from build123d import *

# Parameters (mm, degrees)
SKETCH1_W           = 27
SKETCH1_H           = 12
SKETCH1_R           = 2.1
BOSS_EXTRUDE1_DEPTH = 6
CHAMFER1_SIZE       = 0.5


with BuildPart() as part:
    # Sketch1 → Boss-Extrude1 (new body)
    with BuildSketch(Plane.XY):
        with Locations((13.5, 6)):
            Rectangle(SKETCH1_W, SKETCH1_H)
        with Locations((13.5, 6)):
            Circle(SKETCH1_R, mode=Mode.SUBTRACT)
    extrude(amount=BOSS_EXTRUDE1_DEPTH)

    # Chamfer1
    chamfer1_edges = [part.edges().sort_by_distance(p)[0] for p in [
        (0, 12, 3),
        (27, 12, 3),
        (27, 0, 3),
        (0, 0, 3),
    ]]
    chamfer(chamfer1_edges, length=CHAMFER1_SIZE)


solid = part.part
Design review of the part built by this model. Coordinates are the model's own, in mm. Round coordinates to 2 decimals unless told otherwise and drop trailing zeros. Write each loop counter-clockwise with the first axis right and the second up, starting at its lowest first coordinate (ties: lowest second). Pieces come first, ordered by that corner, then holes. Notation, with made-up numbers: (47.5, -38) - (58.5, -38) arc R34 ccw to (58.5, -1) - close; hole circle Ø6 at (49, 14.5). An arc over 180 degrees is marked (long way). Use a Markdown table: item, result. Add a question column.
1. We need section B-B (z = 0.95). State the section outline as (x, y) points, then the cut area to 3 significant figures.
2. We need section C-C (x = 13.5). State the section outline as (y, z) points.
3. Mouldability with a two-part tool opening along X and no side actions: class faces 1 (the face through (13, 0, 3)), 2 (the face through (0, 6, 3)), 3 (the face through (27, 6, 3)), 4 (the face through (11.952, 7.419, 2.958)) as +X half, -X half, draft (parallel to the pull), parting line (faces both ways), or undercut.
4. Wall thickness on probe 1 along Y at (x, z) = (13.5, 3.55); probe 2 along Y at (x, z) = (14.75, 2.2); probe 3 along X at (y, z) = (7.75, 4.3): over which ranges is each line inside the solid? List them lowest first.
5. Clearance check with a flat-ended pin moving along its axis: pin 1 (4 mm diameter, centred on x = 13.5, y = 6, fed in from -Z). State where the tip first meets the part, or that it passes through.
6. We need section A-A (y = 6). State the section outline as (x, z) points.
Output:
| question | item | result |
|---|---|---|
| 1 | outline | (0, 0.5) - (0.5, 0) - (26.5, 0) - (27, 0.5) - (27, 11.5) - (26.5, 12) - (0.5, 12) - (0, 11.5) - close; hole circle Ø4.2 at (13.5, 6) |
| 1 | area | 310 mm2 |
| 2 | outline | (0, 0) - (3.9, 0) - (3.9, 6) - (0, 6) - close; (8.1, 0) - (12, 0) - (12, 6) - (8.1, 6) - close |
| 3 | face 1 | draft |
| 3 | face 2 | -X half |
| 3 | face 3 | +X half |
| 3 | face 4 | undercut |
| 4 | probe 1 | y = 0 to 3.9, 8.1 to 12 |
| 4 | probe 2 | y = 0 to 4.31, 7.69 to 12 |
| 4 | probe 3 | x = 0 to 12.34, 14.66 to 27 |
| 5 | pin 1 | passes through |
| 6 | outline | (0, 0) - (11.4, 0) - (11.4, 6) - (0, 6) - close; (15.6, 0) - (27, 0) - (27, 6) - (15.6, 6) - close |
